```python
from build123d import *

# Parameters (mm, degrees)
F0_W     = 76.2
F0_H     = 63.5
F1_DEPTH = 19.05
F3_T     = -1.27
F2_R     = 1.5875
F4_DEPTH = 19.05
F4_TAPER = 0.5
F5_W     = 0.22
F5_H     = 10.16
F5_W_2   = 13.75
F5_H_2   = 13.462
F6_DEPTH = 1.27


# Not quite as in the source:
# - a feature names something its author has since deleted; it is built from what else it names


with BuildPart() as f1:
    # F0 (on Front) → F1 (new body)
    with BuildSketch(Plane.XZ):
        with Locations((38.1, 31.75)):
            Rectangle(F0_W, F0_H)
    extrude(amount=F1_DEPTH)

    # F3
    f3_openings = [f1.faces().sort_by_distance(p)[0] for p in [
        (38.1, -19.05, 31.75),
    ]]
    offset(amount=F3_T, openings=f3_openings)

    # F2 (on face) → F4 (join)
    with BuildSketch(Plane.XZ):
        with Locations((59.69, 55.3212)):
            Circle(F2_R)
        with Locations((7.62, 50.2412)):
            Circle(F2_R)
        with Locations((7.62, 22.3012)):
            Circle(F2_R)
        with Locations((58.42, 7.0612)):
            Circle(F2_R)
    extrude(amount=F4_DEPTH, taper=F4_TAPER)

    # F5 (on face) → F6 (cut)
    with BuildSketch(Plane.YZ.offset(76.2)):
        with Locations((-19.16, 50.12)):
            Rectangle(F5_W, F5_H)
        with Locations((-12.175, 50.12)):
            Rectangle(F5_W_2, F5_H)
        with Locations((-19.16, 20.131)):
            Rectangle(F5_W, F5_H_2)
        with Locations((-12.175, 20.131)):
            Rectangle(F5_W_2, F5_H_2)
    extrude(amount=-F6_DEPTH, mode=Mode.SUBTRACT)


solid = f1.part
```
Check sheet for the modelled part. Datum: model origin and axes. Units: mm. A direction names the side the tool comes from. Round coordinates to 2 decimals unless told otherwise and drop trailing zeros. Loops run counter-clockwise (first coordinate to the right, second up) from the corner with the lowest first, then second, coordinate; pieces in that order, holes last. Notation, with made-up numbers: (-34.75, 66) -> (-7.75, 66) arc R26 cw to (-7.75, 85) -> close; hole circle Ø10 at (83, 63.5). An arc over 180 degrees is marked (long way). Answer in a Markdown table with one row per item.
Q1. Sectioned sample at C-C on z = 34. Enter the section's corners in (x, y).
Data:
| item | result |
|---|---|
| outline | (0, -19.05) -> (1.27, -19.05) -> (1.27, -1.27) -> (74.93, -1.27) -> (74.93, -19.05) -> (76.2, -19.05) -> (76.2, 0) -> (0, 0) -> close |
Q2. Sectioned sample at A-A on y = -8.5. Enter the section's corners in (x, z), then the cut area to 3 significant figures.
Data:
| item | result |
|---|---|
| outline | (0, 0) -> (76.2, 0) -> (76.2, 13.4) -> (74.93, 13.4) -> (74.93, 1.27) -> (1.27, 1.27) -> (1.27, 62.23) -> (74.93, 62.23) -> (74.93, 55.2) -> (76.2, 55.2) -> (76.2, 63.5) -> (0, 63.5) -> close; circle Ø3.03 at (7.62, 22.3); circle Ø3.03 at (7.62, 50.24); circle Ø3.03 at (58.42, 7.06); circle Ø3.03 at (59.69, 55.32); (74.93, 26.86) -> (76.2, 26.86) -> (76.2, 45.04) -> (74.93, 45.04) -> close |
| area | 347 mm^2 |
Q3. Set-up check for faces 4 (the face through (8.31, -10.28, 20.97)), 5 (the face through (76.2, -7, 31)): record each of +Z, -Z, +X, -X, +Y, -Y from which the full face is reachable in a straight line by a thin tool's end or side.
Data:
| item | result |
|---|---|
| face 4 | -Y |
| face 5 | +Z, -Z, +X, +Y, -Y |
Q4. Thickness scan on L1, parallel to X at y = -10.5, z = 41.5; L2, parallel to Z at x = 26, y = -8.25; L3, parallel to X at y = -5, z = 22.5. Record the ranges inside material, lowest first.
Data:
| item | result |
|---|---|
| L1 | x = 0 to 1.27, 74.93 to 76.2 |
| L2 | z = 0 to 1.27, 62.23 to 63.5 |
| L3 | x = 0 to 1.27, 6.09 to 9.15, 74.93 to 76.2 |
Q5. Sectioned sample at B-B on x = 19.5. Enter the section's corners in (y, z).
Data:
| item | result |
|---|---|
| outline | (-19.05, 0) -> (0, 0) -> (0, 63.5) -> (-19.05, 63.5) -> (-19.05, 62.23) -> (-1.27, 62.23) -> (-1.27, 1.27) -> (-19.05, 1.27) -> close |
Q6. Sectioned sample at D-D on y = -15.5. Enter the section's corners in (x, z), then the cut area to 3 significant figures.
Data:
| item | result |
|---|---|
| outline | (0, 0) -> (76.2, 0) -> (76.2, 13.4) -> (74.93, 13.4) -> (74.93, 1.27) -> (1.27, 1.27) -> (1.27, 62.23) -> (74.93, 62.23) -> (74.93, 55.2) -> (76.2, 55.2) -> (76.2, 63.5) -> (0, 63.5) -> close; circle Ø2.9 at (7.62, 22.3); circle Ø2.9 at (7.62, 50.24); circle Ø2.9 at (58.42, 7.06); circle Ø2.9 at (59.69, 55.32); (74.93, 26.86) -> (76.2, 26.86) -> (76.2, 45.04) -> (74.93, 45.04) -> close |
| area | 345 mm^2 |
Q7. Release check for a two-part mould opening along X. For faces 1 (the face through (8, -19.05, 50)), 2 (the face through (74.93, -10, 31)), 3 (the face through (0, -9, 31)) record: released by +X, released by -X, zero draft, split by the parting line, or undercut.
Data:
| item | result |
|---|---|
| face 1 | zero draft |
| face 2 | undercut |
| face 3 | released by -X |
Q8. Go/stop test with flat-tipped pins: P1, Ø18.5, axis at x = 23.5, z = 24.5, coming from the -Y side; P2, Ø1.4, axis at x = 75.5, z = 17, coming from the -Y side; P3, Ø10, axis at x = 9, y = -16.5, coming from the -Z side. Record where each tip stops, or that it passes through.
Data:
| item | result |
|---|---|
| P1 | stops at y = -1.27 |
| P2 | stops at y = -5.3 |
| P3 | stops at z = 0 |
